Job drawing, mm, ordinate dimensions from the low corner. One solid piece. A direction names the side the tool comes from. Coordinates: 2 decimals unless noted, no trailing zeros. Write each loop counter-clockwise with the first axis right and the second up, starting at its lowest first coordinate (ties: lowest second). Pieces come first, ordered by that corner, then holes. Notation, with made-up numbers: (1.5, 33.5) - (18.5, 33.5) arc R11 cw to (18.5, 52.5) - close; hole circle Ø10 at (-24, 30.5). An arc over 180 degrees is marked (long way). Use a Markdown table: item, result.
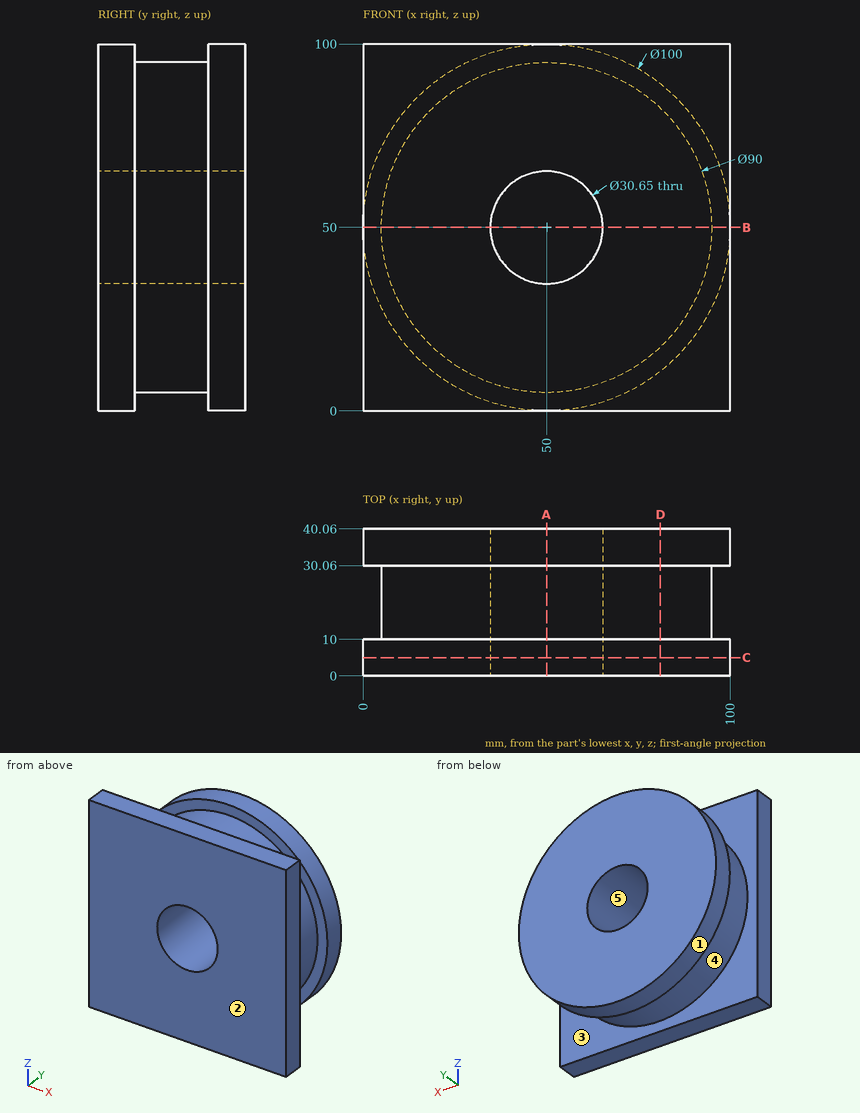
Item 1: Which spindle directions (+Z, -Z, +X, -X, +Y, -Y) get a long thin tool onto all of the face, cutting with end or side? Do the marked faces 4 and 5. Say none if no direction does.
From the geometry:
| item | result |
|---|---|
| face 4 | none |
| face 5 | +Y, -Y |
Item 2: Two-plate mould, pull along Y, no slides. Class the marked faces 1, 2 and 3: pulls with the +Y half, pulls with the -Y half, needs draft (parallel to the pull), parting line crosses it, or undercut.
From the geometry:
| item | result |
|---|---|
| face 1 | needs draft |
| face 2 | pulls with the -Y half |
| face 3 | undercut |
Item 3: Band-saw the part on A-A, the plane x = 50. Give the cut face in (y, z) (3 decimals).
From the geometry:
| item | result |
|---|---|
| outline | (0, 0) - (10, 0) - (10, 5) - (30.06, 5) - (30.06, 0) - (40.06, 0) - (40.06, 34.675) - (0, 34.675) - close; (0, 65.325) - (40.06, 65.325) - (40.06, 100) - (30.06, 100) - (30.06, 95) - (10, 95) - (10, 100) - (0, 100) - close |
Item 4: Band-saw the part on C-C, the plane y = 5. Give the cut face in (x, z) (3 decimals), then the cut area to 3 significant figures.
From the geometry:
| item | result |
|---|---|
| outline | (0, 0) - (100, 0) - (100, 100) - (0, 100) - close; hole circle Ø30.65 at (50, 50) |
| area | 9,260 mm^2 |
Item 5: Band-saw the part on B-B, the plane z = 50. Give the cut face in (x, y) (3 decimals).
From the geometry:
| item | result |
|---|---|
| outline | (0, 0) - (34.675, 0) - (34.675, 40.06) - (0, 40.06) - (0, 30.06) - (5, 30.06) - (5, 10) - (0, 10) - close; (65.325, 0) - (100, 0) - (100, 10) - (95, 10) - (95, 30.06) - (100, 30.06) - (100, 40.06) - (65.325, 40.06) - close |
Item 6: Band-saw the part on D-D, the plane x = 81. Give the cut face in (y, z).
From the geometry:
| item | result |
|---|---|
| outline | (0, 0) - (10, 0) - (10, 17.38) - (30.06, 17.38) - (30.06, 10.77) - (40.06, 10.77) - (40.06, 89.23) - (30.06, 89.23) - (30.06, 82.62) - (10, 82.62) - (10, 100) - (0, 100) - close |
Item 7: Drop flat-ended pins along their axis: P1, Ø12, axis at x = 48.5, z = 53.5, coming from the +Y side; P2, Ø12, axis at x = 76.5, y = 23.5, coming from the -Z side; P3, Ø6, axis at x = 71, y = 25.5, coming from the -Z side; P4, Ø6, axis at y = 19.5, z = 80, coming from the +X side. Give the stop position or say it passes through.
From the geometry:
| item | result |
|---|---|
| P1 | through |
| P2 | z = 9.94 |
| P3 | z = 8.76 |
| P4 | x = 86 |
Item 8: Drill centre lines: probe 1 along X at (y, z) = (29.5, 50) (3 decimals); probe 2 along X at (y, z) = (8.5, 50) (3 decimals); probe 3 along Y at (x, z) = (26.5, 94). Where is each one in solid material? Low to high.
From the geometry:
| item | result |
|---|---|
| probe 1 | 5 to 34.675, 65.325 to 95 |
| probe 2 | 0 to 34.675, 65.325 to 100 |
| probe 3 | 0 to 10, 30.06 to 40.06 |
